Could you check a few things on this model? Use its own coordinates, in mm. A direction names the side the tool comes from. Give positions to 0.01 mm unless a question says otherwise; leave off trailing zeros. Order: outer loops, then holes, each group sorted by start corner. A loop starts at its lowest first (then second) coordinate and runs counter-clockwise, first axis right, second up. Notation, with made-up numbers: (88.5, 75.5) - (111.5, 75.5) arc R18 ccw to (111.5, 84.5) - close; hole circle Ø6 at (78.25, 78). An arc over 180 degrees is marked (long way). Put each result on its own line as item: value.
from build123d import *

# Parameters (mm, degrees)
SKETCH_R      = 7.25
SKETCH_R_2    = 5.2
PAD_DEPTH     = 6
SKETCH001_R   = 7.25
PAD001_DEPTH  = 3
FILLET_R      = 2
FILLET001_R   = 0.3
SKETCH002_R   = 5.2
SKETCH002_R_2 = 4.1
PAD002_DEPTH  = 3.4


with BuildPart() as part:
    # Sketch → Pad (new body)
    with BuildSketch(Plane.XY):
        Circle(SKETCH_R)
        Circle(SKETCH_R_2, mode=Mode.SUBTRACT)
    extrude(amount=PAD_DEPTH)

    # Sketch001 (on Face4 of Pad) → Pad001 (join)
    with BuildSketch(Plane.XY.offset(6)):
        Circle(SKETCH001_R)
    extrude(amount=PAD001_DEPTH)

    # Fillet
    fillet_edges = [part.edges().sort_by_distance(p)[0] for p in [
        (-7.25, 0, 9),
    ]]
    fillet(fillet_edges, radius=FILLET_R)

    # Fillet001
    fillet001_edges = [part.edges().sort_by_distance(p)[0] for p in [
        (-5.2, 0, 0),
    ]]
    fillet(fillet001_edges, radius=FILLET001_R)

    # Sketch002 (on Face6 of Fillet001) → Pad002 (join)
    with BuildSketch(Plane(origin=(0, 0, 6), x_dir=(1, 0, 0), z_dir=(0, 0, -1))):
        Circle(SKETCH002_R)
        Circle(SKETCH002_R_2, mode=Mode.SUBTRACT)
    extrude(amount=PAD002_DEPTH)


solid = part.part
1) If I drill on line 1 (Y direction, x = 0, z = 4.25); line 2 (Y direction, x = 0, z = 0.85); line 3 (X direction, y = 3, z = 2.75), over which ranges is the centre line in solid material (lowest first)? Write a range as [from, to].
Filled in:
line 1: y = [-7.25, -4.1], [4.1, 7.25]
line 2: y = [-7.25, -5.2], [5.2, 7.25]
line 3: x = [-6.6, -2.79], [2.79, 6.6]
2) Suppose I cut it at A-A, the plane y = 0. List the corners of the cut face in (x, z) for me.
Filled in:
outline: (-7.25, 0) - (-5.5, 0) arc R0.3 ccw to (-5.2, 0.3) - (-5.2, 2.6) - (-4.1, 2.6) - (-4.1, 6) - (4.1, 6) - (4.1, 2.6) - (5.2, 2.6) - (5.2, 0.3) arc R0.3 ccw to (5.5, 0) - (7.25, 0) - (7.25, 7) arc R2 ccw to (5.25, 9) - (-5.25, 9) arc R2 ccw to (-7.25, 7) - close
3) Suppose I cut it at D-D, the plane z = 5.75. List the corners of the cut face in (x, y) for me, and give its area (3 significant figures).
Filled in:
outline: circle Ø14.5 at (0, 0); hole circle Ø8.2 at (0, 0)
area: 112 mm^2
4) Suppose I cut it at B-B, the plane z = 1.25. List the corners of the cut face in (x, y) for me.
Filled in:
outline: circle Ø14.5 at (0, 0); hole circle Ø10.4 at (0, 0)
5) We'd pull the mould along X, two halves only. Please class faces 1 (the cylindrical face through (3.35, -6.43, 3.45)), 2 (the cylindrical face through (-0.534, -4.065, 4.324)), 3 (the flat face through (3, 5, 0)): pulls with the +X half, pulls with the -X half, needs draft (parallel to the pull), parting line crosses it, or undercut.
Filled in:
face 1: parting line crosses it
face 2: undercut
face 3: needs draft
6) Which directions (+Z, -Z, +X, -X, +Y, -Y) give clear straight access to the entire face, cutting with the end or side of a thin tool? Please do faces 4 (the flat face through (0, 0, 9)), 5 (the flat face through (4, -2, 2.6)).
Filled in:
face 4: +Z, +X, -X, +Y, -Y
face 5: -Z
7) I'm going to push flat-ended pins straight in: pin 1 (2 mm diameter, centred on x = 5, z = 6.5, fed in from +Y); pin 2 (4 mm diameter, centred on x = -2.5, y = 1.5, fed in from -Z); pin 3 (3 mm diameter, centred on x = -0.5, y = -1.5, fed in from -Z). Where does each tip first touch, or does it pass through?
Filled in:
pin 1: stops at y = 6.05
pin 2: stops at z = 2.6
pin 3: stops at z = 6
